Verification items for the finished model (mm, model axes). A direction names the side the tool comes from. Give positions to 0.01 mm unless a question says otherwise; leave off trailing zeros. Write each loop counter-clockwise with the first axis right and the second up, starting at its lowest first coordinate (ties: lowest second). Pieces come first, ordered by that corner, then holes. Notation, with made-up numbers: (-27.5, 61) - (8.5, 61) arc R25 ccw to (8.5, 78) - close; hole circle Ø1 at (78.5, 12.5). An arc over 180 degrees is marked (long way). Put each result on its own line as item: value.
from build123d import *

# Parameters (mm, degrees)
SKETCH1_R                   = 25.4
BOSS_EXTRUDE1_DEPTH         = 152.4
SKETCH3_W                   = 25.4
SKETCH3_H                   = 88.9
CUT_EXTRUDE1_DEPTH          = 102.6
CUT_EXTRUDE1_DEPTH_BACK     = 102.6
F_1_4_0_25_DIAMETER_HOLE1_D = 6.35
SKETCH4_W                   = 25.4
SKETCH4_H                   = 101.6
CUT_EXTRUDE2_DEPTH          = 13.7
SKETCH7_W                   = 203.2
SKETCH7_H                   = 210.309489201
BOSS_EXTRUDE2_DEPTH         = 152.4
CUT_EXTRUDE3_DEPTH          = 204.2


with BuildPart() as part:
    # Sketch1 → Boss-Extrude1 (new body)
    with BuildSketch(Plane.XY):
        with BuildLine():
            Line((-101.6, -50.8), (101.6, -50.8))
            Line((101.6, -50.8), (101.6, -38.1))
            Line((101.6, -38.1), (76.2, -38.1))
            Line((76.2, -38.1), (76.2, -12.7))
            ThreePointArc((76.2, -12.7), (57.601280605, 32.201280605), (12.7, 50.8))
            Line((12.7, 50.8), (-12.7, 50.8))
            ThreePointArc((-12.7, 50.8), (-57.601280605, 32.201280605), (-76.2, -12.7))
            Line((-76.2, -12.7), (-76.2, -38.1))
            Line((-76.2, -38.1), (-101.6, -38.1))
            Line((-101.6, -38.1), (-101.6, -50.8))
        make_face()
        Circle(SKETCH1_R, mode=Mode.SUBTRACT)
    extrude(amount=BOSS_EXTRUDE1_DEPTH)

    # Sketch3 → Cut-Extrude1 (cut, two sides)
    with BuildSketch(Plane(origin=(0, 0, 0), x_dir=(0, 0, -1), z_dir=(1, 0, 0))) as cut_extrude1_sk:
        with Locations((-114.3, 6.35)):
            Rectangle(SKETCH3_W, SKETCH3_H)
        with Locations((-38.1, 6.35)):
            Rectangle(SKETCH3_W, SKETCH3_H)
    extrude(amount=CUT_EXTRUDE1_DEPTH, mode=Mode.SUBTRACT)
    extrude(cut_extrude1_sk.sketch, amount=-CUT_EXTRUDE1_DEPTH_BACK, mode=Mode.SUBTRACT)

    # 1/4 (0.25) Diameter Hole1 (through all)
    with Locations(Plane(origin=(0, -38.1, 0), x_dir=(1, 0, 0), z_dir=(0, 1, 0))):
        with Locations((-88.9, -12.7), (-88.9, -139.7), (88.9, -12.7), (88.9, -139.7)):
            Hole(F_1_4_0_25_DIAMETER_HOLE1_D / 2)

    # Sketch4 → Cut-Extrude2 (cut, through all)
    with BuildSketch(Plane(origin=(0, -38.1, 0), x_dir=(1, 0, 0), z_dir=(0, 1, 0))):
        with Locations((-88.9, -76.2)):
            Rectangle(SKETCH4_W, SKETCH4_H)
        with Locations((88.9, -76.2)):
            Rectangle(SKETCH4_W, SKETCH4_H)
    extrude(amount=-CUT_EXTRUDE2_DEPTH, mode=Mode.SUBTRACT)

    # Sketch7 → Boss-Extrude2 (add)
    with BuildSketch(Plane(origin=(0, 0, 0), x_dir=(-1, 0, 0), z_dir=(0, 0, -1))):
        with Locations((0, -155.954744601)):
            Rectangle(SKETCH7_W, SKETCH7_H)
    extrude(amount=-BOSS_EXTRUDE2_DEPTH)

    # Sketch8 → Cut-Extrude3 (cut, through all)
    with BuildSketch(Plane(origin=(101.6, 0, 0), x_dir=(0, 0, -1), z_dir=(1, 0, 0))):
        with BuildLine():
            Line((-152.4, -261.109489201), (0, -261.109489201))
            ThreePointArc((0, -261.109489201), (-76.2, -258.687695415), (-152.4, -261.109489201))
        make_face()
    extrude(amount=-CUT_EXTRUDE3_DEPTH, mode=Mode.SUBTRACT)


solid = part.part
Q1. Section check C-C, the plane z = 82.5. Record the cut outline in (x, y), plus the area to 3 significant figures.
Answers follow:
outline: (-101.6, -258.7) - (101.6, -258.7) - (101.6, -50.8) - (76.2, -50.8) - (76.2, -12.7) arc R63.5 ccw to (12.7, 50.8) - (-12.7, 50.8) arc R63.5 ccw to (-76.2, -12.7) - (-76.2, -50.8) - (-101.6, -50.8) - close; hole circle Ø50.8 at (0, 0)
area: 54,000 mm2
Q2. Set-up check for faces 1 (the face through (-76.2, -25, 13)), 2 (the face through (-89, -44, 127)), 3 (the face through (89, -44, 127)): record each of +Z, -Z, +X, -X, +Y, -Y from which the full face is reachable in a straight line by a thin tool's end or side.
Answers follow:
face 1: +Z, -Z, -X, +Y
face 2: -X, +Y
face 3: +X, +Y
Q3. Section check B-B, the plane y = 0. Record the cut outline in (x, z).
Answers follow:
outline: (-74.92, 0) - (-25.4, 0) - (-25.4, 25.4) - (-74.92, 25.4) - close; (-74.92, 50.8) - (-25.4, 50.8) - (-25.4, 101.6) - (-74.92, 101.6) - close; (-74.92, 127) - (-25.4, 127) - (-25.4, 152.4) - (-74.92, 152.4) - close; (25.4, 0) - (74.92, 0) - (74.92, 25.4) - (25.4, 25.4) - close; (25.4, 50.8) - (74.92, 50.8) - (74.92, 101.6) - (25.4, 101.6) - close; (25.4, 127) - (74.92, 127) - (74.92, 152.4) - (25.4, 152.4) - close
Q4. Release check for a two-part mould opening along Y. For faces 4 (the face through (-5.506, -24.796, 12.522)), 5 (the face through (76.2, -36, 77)), 6 (the face through (89, -50.8, 13)) record: released by +Y, released by -Y, zero draft, split by the parting line, or undercut.
Answers follow:
face 4: undercut
face 5: zero draft
face 6: released by +Y
Q5. Go/stop test with flat-tipped pins: pin 1 Ø12.5 at (x, z) = (11.5, 116) entering from +Y; pin 2 Ø1.9 at (x, z) = (89.5, 139) entering from +Y; pin 3 Ø20.5 at (y, z) = (-22.5, 12.5) entering from +X. Record where each tip stops, or that it passes through.
Answers follow:
pin 1: stops at y = -38.1
pin 2: stops at y = -50.8
pin 3: stops at x = 76.2
Q6. Section check A-A, the plane x = 0. Record the cut outline in (y, z).
Answers follow:
outline: (-261.11, 0) - (-25.4, 0) - (-25.4, 25.4) - (-38.1, 25.4) - (-38.1, 50.8) - (-25.4, 50.8) - (-25.4, 101.6) - (-38.1, 101.6) - (-38.1, 127) - (-25.4, 127) - (-25.4, 152.4) - (-261.11, 152.4) arc R1200 cw to start; (25.4, 0) - (50.8, 0) - (50.8, 25.4) - (25.4, 25.4) - close; (25.4, 50.8) - (50.8, 50.8) - (50.8, 101.6) - (25.4, 101.6) - close; (25.4, 127) - (50.8, 127) - (50.8, 152.4) - (25.4, 152.4) - close
Q7. Section check D-D, the plane x = 44. Record the cut outline in (y, z).
Answers follow:
outline: (-261.11, 0) - (42.55, 0) - (42.55, 25.4) - (-38.1, 25.4) - (-38.1, 50.8) - (42.55, 50.8) - (42.55, 101.6) - (-38.1, 101.6) - (-38.1, 127) - (42.55, 127) - (42.55, 152.4) - (-261.11, 152.4) arc R1200 cw to start
Q8. Scan lines: line 1 along X through (y, z) = (-42.5, 12.7) (3 decimals); line 2 along Z through (x, y) = (-33, 6.5); line 3 along Z through (x, y) = (88.9, -48) (3 decimals). Record each from-to range of solid material in increasing order.
Answers follow:
line 1: x = -101.6 to -92.075, -85.725 to 85.725, 92.075 to 101.6
line 2: z = 0 to 25.4, 50.8 to 101.6, 127 to 152.4
line 3: z = 0 to 9.525, 15.875 to 25.4, 127 to 136.525, 142.875 to 152.4
